```python
from build123d import *

# Parameters (mm, degrees)
SKETCH1_R           = 3.175
BOSS_EXTRUDE1_DEPTH = 19
SKETCH2_W           = 28
SKETCH2_H           = 12.7
BOSS_EXTRUDE2_DEPTH = 3.175
BOSS_EXTRUDE3_DEPTH = 6.35
FILLET1_R           = 2.54
FILLET2_R           = 2.54


with BuildPart() as part:
    # Sketch1 → Boss-Extrude1 (new, symmetric)
    with BuildSketch(Plane(origin=(0, 0, 0), x_dir=(1, 0, 0), z_dir=(0, 1, 0))):
        with Locations(Location((0, 0, 0), (0, 0, 270))):
            Circle(SKETCH1_R)
    extrude(amount=BOSS_EXTRUDE1_DEPTH, both=True)

    # Sketch2 → Boss-Extrude2 (add)
    with BuildSketch(Plane.XZ.offset(19)):
        with Locations((-5.11, 0)):
            Rectangle(SKETCH2_W, SKETCH2_H)
    extrude(amount=-BOSS_EXTRUDE2_DEPTH)

    # Sketch3 → Boss-Extrude3 (add)
    with BuildSketch(Plane.XZ.offset(19)):
        Polygon((-13.395, -6.35), (-13.395, 15.65), (-19.745, 15.65), (-19.745, 35.65), (-0.695, 35.65), (-0.695, 15.65), (-7.045, 15.65), (-7.045, -6.35), align=None)
    extrude(amount=BOSS_EXTRUDE3_DEPTH)

    # Fillet1
    fillet1_edges = [part.edges().sort_by_distance(p)[0] for p in [
        (-13.395, -25.35, 4.65),
        (-16.57, -25.35, 15.65),
        (-3.87, -25.35, 15.65),
        (-7.045, -25.35, 4.65),
        (-10.22, -25.35, -6.35),
        (-0.695, -22.175, 15.65),
        (-0.695, -25.35, 25.65),
        (-0.695, -19, 25.65),
        (-0.695, -22.175, 35.65),
        (-10.22, -25.35, 35.65),
        (-10.22, -19, 35.65),
        (-19.745, -22.175, 35.65),
        (-19.745, -25.35, 25.65),
        (-19.745, -22.175, 15.65),
        (-19.745, -19, 25.65),
        (-3.87, -19, 15.65),
        (-16.57, -19, 15.65),
        (-7.045, -19, 11),
        (-13.395, -19, 11),
        (-7.045, -22.175, -6.35),
        (-13.395, -22.175, -6.35),
    ]]
    fillet(fillet1_edges, radius=FILLET1_R)

    # Fillet2
    # the kernel refuses this fillet: 2.54 mm, written as the material it adds along each edge
    with BuildSketch(Plane(origin=(-9.585, -19, -3.81), x_dir=(-0.5976672776328281, 0, 0.8017442392976477), z_dir=(0.8017442392976477, 0, 0.5976672776328281))) as fillet2_piece_1_section:
        with BuildLine():
            CenterArc((2.54 + FILLET2_R, FILLET2_R), FILLET2_R, 180, 90)
            Line((2.54, FILLET2_R), (2.54, 0))
            Line((2.54, 0), (2.54 + FILLET2_R, 0))
        make_face()
    fillet2_piece_1 = revolve(axis=Axis((-9.585, -19, -3.81), (0, -1, 0)), revolution_arc=233.296989237, mode=Mode.PRIVATE)
    fillet2_piece_1 = split(fillet2_piece_1, bisect_by=Plane(origin=(-13.679769983, -19.079873008, -6.35), z_dir=(0, 0, 1)), keep=Keep.TOP, mode=Mode.PRIVATE)
    add(fillet2_piece_1)
    with BuildSketch(Plane(origin=(-10.855, -19, -3.81), x_dir=(0.5976672776328281, 0, 0.8017442392976477), z_dir=(-0.8017442392976477, 0, 0.5976672776328281))) as fillet2_piece_2_section:
        with BuildLine():
            CenterArc((2.54 + FILLET2_R, -FILLET2_R), FILLET2_R, 90, 90)
            Line((2.54, -FILLET2_R), (2.54, 0))
            Line((2.54, 0), (2.54 + FILLET2_R, 0))
        make_face()
    fillet2_piece_2 = revolve(axis=Axis((-10.855, -19, -3.81), (0, 1, 0)), revolution_arc=233.296989237, mode=Mode.PRIVATE)
    fillet2_piece_2 = split(fillet2_piece_2, bisect_by=Plane(origin=(-6.760230017, -19.079873008, -6.35), z_dir=(0, 0, 1)), keep=Keep.TOP, mode=Mode.PRIVATE)
    add(fillet2_piece_2)
    with BuildSketch(Plane(origin=(-7.045, -19, 6.35), x_dir=(1, 0, 0), z_dir=(0, 0, -1)), Plane(origin=(-13.395, -19, -3.81), x_dir=(-1, 0, 0), z_dir=(0, 0, 1))) as fillet2_piece_3:
        with BuildLine():
            CenterArc((FILLET2_R, FILLET2_R), FILLET2_R, 180, 90)
            Line((0, FILLET2_R), (0, 0))
            Line((0, 0), (FILLET2_R, 0))
        make_face()
    extrude(amount=10.16)


solid = part.part
```
Check sheet for the modelled part. Datum: model origin and axes. Units: mm. A direction names the side the tool comes from. Round coordinates to 2 decimals unless told otherwise and drop trailing zeros. Order: outer loops, then holes, each group sorted by start corner. A loop starts at its lowest first (then second) coordinate and runs counter-clockwise, first axis right, second up. Notation, with made-up numbers: (45.5, 83) -> (71.5, 83) arc R24 cw to (71.5, 101) -> close; hole circle Ø1 at (-1, -29.5). An arc over 180 degrees is marked (long way). One line per item, written item: value. Start each with the question number.
Q1. Thickness scan on line 1 (X direction, y = -22.5, z = 26) (3 decimals); line 2 (X direction, y = -21.5, z = 8.5); line 3 (Y direction, x = -12.75, z = 31). Record the ranges inside material, lowest first.
Q2. Set-up check for faces 1 (the face through (-18, -19, 0)), 2 (the face through (-7.045, -22, 6)), 3 (the face through (-10.229, -24.586, -5.626)): record each of +Z, -Z, +X, -X, +Y, -Y from which the full face is reachable in a straight line by a thin tool's end or side.
Q3. Cross-section at D-D (z = 0). Record the boundary of the cut face in (x, y) (3 decimals), and give its area (3 significant figures).
Q4. Cross-section at B-B (x = 0). Record the boundary of the cut face in (y, z) (3 decimals), and give its area (3 significant figures).
Q5. Gauge pin test, flat ends, axial feed: pin 1 Ø10 at (x, z) = (-5, 2) entering from +Y; pin 2 Ø1 at (x, z) = (-15.5, 13) entering from -Y; pin 3 Ø0.6 at (y, z) = (-22, 26) entering from +X (3 decimals); pin 4 Ø15.5 at (x, z) = (-8, 24) entering from +Y. Record the tip position at first contact, or that the pin passes through.
Q6. Cross-section at C-C (y = 11). Record the boundary of the cut face in (x, z) (3 decimals), and give its area (3 significant figures).
Q7. Cross-section at A-A (z = 10.5). Record the boundary of the cut face in (x, y) (3 decimals), and give its area (3 significant figures).
Completed:
1. line 1: x = -19.745 to -0.695
1. line 2: x = -13.39 to -7.05
1. line 3: y = -25.35 to -19
2. face 1: -Z, -X, -Y
2. face 2: -Z, +X, -Y
2. face 3: -Z, +X, -X, -Y
3. outline: (-19.11, -19) -> (-15.935, -19) arc R2.54 cw to (-13.395, -21.54) -> (-13.395, -22.81) arc R2.54 ccw to (-10.855, -25.35) -> (-9.585, -25.35) arc R2.54 ccw to (-7.045, -22.81) -> (-7.045, -21.54) arc R2.54 cw to (-4.505, -19) -> (8.89, -19) -> (8.89, -15.825) -> (3.175, -15.825) -> (3.175, 19) -> (-3.175, 19) -> (-3.175, -15.825) -> (-19.11, -15.825) -> close
3. area: 350 mm²
4. outline: (-19, -6.35) -> (-15.825, -6.35) -> (-15.825, -3.175) -> (19, -3.175) -> (19, 3.175) -> (-15.825, 3.175) -> (-15.825, 6.35) -> (-19, 6.35) -> close
4. area: 261 mm²
5. pin 1: stops at y = 19
5. pin 2: passes through
5. pin 3: stops at x = -0.695
5. pin 4: stops at y = -19
6. outline: circle Ø6.35 at (0, 0)
6. area: 31.7 mm²
7. outline: (-13.395, -22.81) arc R2.54 ccw to (-10.855, -25.35) -> (-9.585, -25.35) arc R2.54 ccw to (-7.045, -22.81) -> (-7.045, -21.54) arc R2.54 ccw to (-9.585, -19) -> (-10.855, -19) arc R2.54 ccw to (-13.395, -21.54) -> close
7. area: 34.8 mm²
